Could you check a few things on this model? Use its own coordinates, in mm. A direction names the side the tool comes from. Round coordinates to 2 decimals unless told otherwise and drop trailing zeros. Loops run counter-clockwise (first coordinate to the right, second up) from the corner with the lowest first, then second, coordinate; pieces in that order, holes last. Notation, with made-up numbers: (-29, -25.5) -> (8, -25.5) arc R20 cw to (8, 6.5) -> close; hole circle Ø6 at (-9.5, 86.5). An arc over 180 degrees is marked (long way). One line per item, written item: value.
from build123d import *

# Parameters (mm, degrees)
F0_W     = 45.212
F0_H     = 63.5
F1_DEPTH = 1.524
F2_W     = 45.212
F2_H     = 63.5
F2_W_2   = 43.18
F2_H_2   = 59.435986
F3_DEPTH = 43.434
F4_R     = 1.27


with BuildPart() as f1:
    # F0 (on Top) → F1 (new body)
    with BuildSketch(Plane.XY):
        Rectangle(F0_W, F0_H)
    extrude(amount=F1_DEPTH)

    # F2 (on face) → F3 (join)
    with BuildSketch(Plane.XY.offset(1.524)):
        Rectangle(F2_W, F2_H)
        with Locations((0, 0.413703)):
            Rectangle(F2_W_2, F2_H_2, mode=Mode.SUBTRACT)
    extrude(amount=F3_DEPTH)

    # F4
    f4_edges = [f1.edges().sort_by_distance(p)[0] for p in [
        (0, 31.75, 0),
        (-22.606, 0, 0),
        (0, -31.75, 0),
        (22.606, 0, 0),
    ]]
    fillet(f4_edges, radius=F4_R)


solid = f1.part
(1) If I drill on L1, parallel to X at y = 0.5, z = 19.5; L2, parallel to Y at x = -19.5, z = 39.5; L3, parallel to Z at x = -20.5, y = -24.5, over which ranges is the centre line in solid material (lowest first)?
Recorded:
L1: -22.61 to -21.59, 21.59 to 22.61
L2: -31.75 to -29.3, 30.13 to 31.75
L3: 0 to 1.52
(2) For faces 5 (the face through (22.606, 0, 23)), 6 (the face through (0, 1, 1.524)), which set-ups out of +Z, -Z, +X, -X, +Y, -Y let a thin tool reach every point of the face, with its end or its side?
Recorded:
face 5: +Z, -Z, +X, +Y, -Y
face 6: +Z
(3) I'm going to push a flat-ended pin straight in: pin 1 Ø13 at (x, y) = (-1.5, -10.5) entering from +Z. Where does the tip first touch, or does it pass through?
Recorded:
pin 1: z = 1.52
(4) If we section it at C-C, the plane y = -26: Please give me the cut outline in (x, z).
Recorded:
outline: (-22.61, 1.27) arc R1.27 ccw to (-21.34, 0) -> (21.34, 0) arc R1.27 ccw to (22.61, 1.27) -> (22.61, 44.96) -> (21.59, 44.96) -> (21.59, 1.52) -> (-21.59, 1.52) -> (-21.59, 44.96) -> (-22.61, 44.96) -> close
(5) If we section it at A-A, the plane z = 42.5: Please give me the cut outline in (x, y), then the cut area to 3 significant figures.
Recorded:
outline: (-22.61, -31.75) -> (22.61, -31.75) -> (22.61, 31.75) -> (-22.61, 31.75) -> close; hole (-21.59, -29.3) -> (21.59, -29.3) -> (21.59, 30.13) -> (-21.59, 30.13) -> close
area: 305 mm²
(6) Thinking about a two-plate mould opening in X: for faces 1 (the face through (-22.606, 0, 23)), 2 (the face through (21.59, 0, 23)), 3 (the face through (-21.59, 0, 23)), 4 (the face through (0, -31.75, 23)), which applies, released by +X, released by -X, zero draft, split by the parting line, or undercut?
Recorded:
face 1: released by -X
face 2: undercut
face 3: undercut
face 4: zero draft
(7) If we section it at B-B, the plane x = 11: Please give me the cut outline in (y, z), then the cut area to 3 significant figures.
Recorded:
outline: (-31.75, 1.27) arc R1.27 ccw to (-30.48, 0) -> (30.48, 0) arc R1.27 ccw to (31.75, 1.27) -> (31.75, 44.96) -> (30.13, 44.96) -> (30.13, 1.52) -> (-29.3, 1.52) -> (-29.3, 44.96) -> (-31.75, 44.96) -> close
area: 273 mm²
